CAD build for the part. Positions are in the model's coordinates, mm. A direction names the side the tool comes from. Give positions to 0.01 mm unless a question says otherwise; leave off trailing zeros. Loops run counter-clockwise (first coordinate to the right, second up) from the corner with the lowest first, then second, coordinate; pieces in that order, holes last.
Item 1: Saw through at B-B on x = 354. Give the cut face in (y, z).
Item 2: Saw through at A-A on x = 43.5. Give the cut face in (y, z), plus the area to 3 significant figures.
Item 3: Saw through at C-C on x = 228. Give the cut face in (y, z), plus the area to 3 significant figures.
Item 4: Probe probe 1 along Y at (x, z) = (161.5, 0); probe 2 along Z at (x, y) = (354, -10); probe 3 along Y at (x, z) = (109, 1). List the from-to ranges inside material, lowest first.
Item 5: Which spindle directions (+Z, -Z, +X, -X, +Y, -Y) get a long thin tool onto all of the face, cutting with end or side? Do faces 5 (the flat face through (-7, -15, 18)), 6 (the cylindrical face through (328, 0, -8)), 7 (the flat face through (-9, 20, -4)), 8 (the flat face through (345, -20, -4)). Say none if no direction does.
Item 6: Mould opens along Y. For faces 1 (the flat face through (218, -10, -25)), 2 (the flat face through (345, 20, -4)), 3 (the conical face through (321.625, -19.662, -4.366)), 4 (the cylindrical face through (125, 8, 25)) say: released by +Y, released by -Y, zero draft, split by the parting line, or undercut.
Item 7: Drop flat-ended pins along their axis: P1, Ø12, axis at y = 3, z = 11.5, coming from the -X side; P2, Ø3, axis at y = -17.5, z = 4, coming from the -X side; P3, Ø8, axis at x = 223.5, y = 1.5, coming from the +Z side; P4, Ø8, axis at x = 45, y = -3.5, coming from the -Z side. Give the stop position or say it passes through.
from build123d import *

# Parameters (mm, degrees)
F0_W     = 188.5
F0_H     = 4
F0_W_2   = 12
F0_H_2   = 2
F0_W_3   = 11
F0_H_3   = 8
F0_W_4   = 96
F2_R     = 22
F2_R_2   = 19
F3_DEPTH = 15
F4_R     = 19
F4_R_2   = 9.5
F5_DEPTH = 20


with BuildPart() as f1:
    # F0 (on Front) → F1 (revolve)
    with BuildSketch(Plane.XZ):
        Polygon((28, 6.5574385243), (28, 0), (29.5, 0), (29.5, 4), (29.5, 26.25), (218, 26.25), (218, 27.75), (28, 27.75), align=None)
        with BuildLine():
            ThreePointArc((21, 6.5574385243), (21.7485631709, 3.3166247904), (22, 0))
            Line((22, 0), (28, 0))
            Line((28, 0), (28, 6.5574385243))
            Line((28, 6.5574385243), (21, 6.5574385243))
        make_face()
        with Locations((123.75, 2)):
            Rectangle(F0_W, F0_H)
        Polygon((314, 4), (314, 0), (316, 0), (316, 22.25), (218, 22.25), (218, 20.25), (314, 20.25), align=None)
        with Locations((212, 21.25)):
            Rectangle(F0_W_2, F0_H_2)
        Polygon((316, 22.25), (316, 0), (322, 0), (322, 8), (322, 20), align=None)
        with Locations((327.5, 4)):
            Rectangle(F0_W_3, F0_H_3)
        with Locations((266, 2)):
            Rectangle(F0_W_4, F0_H)
    revolve(axis=Axis((171.75, 0, 0), (-1, 0, 0)))

    # F2 (on Front) → F3 (join, symmetric)
    with BuildSketch(Plane.XZ):
        Circle(F2_R)
        Circle(F2_R_2, mode=Mode.SUBTRACT)
        with BuildLine():
            ThreePointArc((376, 0), (357.3166247904, 21.7485631709), (333, 6.5574385243))
            Line((333, 6.5574385243), (333, -6.5574385243))
            ThreePointArc((333, -6.5574385243), (357.3166247904, -21.7485631709), (376, 0))
        make_face()
        with Locations((354, 0)):
            Circle(F2_R_2, mode=Mode.SUBTRACT)
        with BuildLine():
            Line((333, -6.5574385243), (333, 6.5574385243))
            ThreePointArc((333, 6.5574385243), (332, 0), (333, -6.5574385243))
        make_face()
    extrude(amount=F3_DEPTH, both=True)

    # F4 (on Front) → F5 (join, symmetric)
    with BuildSketch(Plane.XZ):
        Circle(F4_R)
        Circle(F4_R_2, mode=Mode.SUBTRACT)
        with Locations((354, 0)):
            Circle(F4_R)
        with Locations((354, 0)):
            Circle(F4_R_2, mode=Mode.SUBTRACT)
    extrude(amount=F5_DEPTH, both=True)


solid = f1.part
Results below:
1. outline: (-20, -19) - (-15, -19) - (-15, -22) - (15, -22) - (15, -19) - (20, -19) - (20, -9.5) - (-20, -9.5) - close; (-20, 9.5) - (20, 9.5) - (20, 19) - (15, 19) - (15, 22) - (-15, 22) - (-15, 19) - (-20, 19) - close
2. outline: circle Ø55.5 at (0, 0); circle Ø8 at (0, 0); hole circle Ø52.5 at (0, 0)
2. area: 305 mm2
3. outline: circle Ø44.5 at (0, 0); circle Ø8 at (0, 0); hole circle Ø40.5 at (0, 0)
3. area: 317 mm2
4. probe 1: y = -27.75 to -26.25, -4 to 4, 26.25 to 27.75
4. probe 2: z = -22 to -9.5, 9.5 to 22
4. probe 3: y = -27.73 to -26.23, -3.87 to 3.87, 26.23 to 27.73
5. face 5: -Y
5. face 6: none
5. face 7: +Z, -Z, -X, +Y
5. face 8: +Z, -Z, +X, -Y
6. face 1: zero draft
6. face 2: released by +Y
6. face 3: split by the parting line
6. face 4: undercut
7. P1: stops at x = -21.3
7. P2: stops at x = -18.83
7. P3: stops at z = 22.25
7. P4: stops at z = -27.75
